Input: part model. Units: mm. Frame: model coordinates. Coordinates: 2 decimals unless noted, no trailing zeros. Order: outer loops, then holes, each group sorted by start corner. A loop starts at its lowest first (then second) coordinate and runs counter-clockwise, first axis right, second up. Notation, with made-up numbers: (-32, 51) - (21, 51) arc R24 cw to (21, 79) - close; hole circle Ø9 at (43, 39). An arc over 180 degrees is marked (long way). One line per question, with ' | ' between items.
from build123d import *


with BuildPart() as part:
    # Skizze1 → Rotation1 (revolve)
    with BuildSketch(Plane(origin=(0, 0, 0), x_dir=(0, 0, -1), z_dir=(1, 0, 0))):
        with BuildLine():
            Line((0, 0), (0, 10.5))
            ThreePointArc((0, 10.5), (0.292893219, 11.207106781), (1, 11.5))
            Line((1, 11.5), (42, 11.5))
            ThreePointArc((42, 11.5), (42.707106781, 11.207106781), (43, 10.5))
            Line((43, 10.5), (43, 8))
            Line((43, 8), (42.5, 7.5))
            Line((42.5, 7.5), (42.5, 5))
            Line((42.5, 5), (43, 4.5))
            Line((43, 4.5), (43, 0))
            Line((43, 0), (0, 0))
        make_face()
    revolve(axis=Axis((0, 0, 0), (0, 0, -1)))


solid = part.part
Item 1: Section A-A on z = -20.5. Return the cut outline in (x, y).
Data:
outline: circle Ø23 at (0, 0)
Item 2: Contact query for flat-ended pins moving along their axis: P1, Ø1, axis at x = 8, z = -37.5, coming from the +Y side; P2, Ø2, axis at y = 2.5, z = -8, coming from the -X side; P3, Ø12, axis at x = 9, z = -25.5, coming from the -Y side. Output: stop coordinate, or through.
Data:
P1: y = 8.72 | P2: x = -11.4 | P3: y = -11.1
Item 3: Ray query, line 1 (Z direction, x = 6.5, y = 0.5); line 2 (Y direction, x = 8.25, z = -27); line 3 (X direction, y = 0.5, z = -35). Return the intervals inside material, ascending.
Data:
line 1: -42.5 to 0 | line 2: -8.01 to 8.01 | line 3: -11.49 to 11.49
Item 4: Draft query along X for faces 1 (the face through (-5, 2, -42.5)), 2 (the face through (11.4, -1.5, -21.8)), 3 (the face through (0, 0, 0)). Return one class per face: released by +X, released by -X, zero draft, split by the parting line, or undercut.
Data:
face 1: undercut | face 2: split by the parting line | face 3: zero draft
